For this review, take the finished solid that the model builds, in its own axes (mm). A direction names the side the tool comes from. Round coordinates to 2 decimals unless told otherwise and drop trailing zeros. Write each loop counter-clockwise with the first axis right and the second up, starting at its lowest first coordinate (ties: lowest second). Pieces come first, ordered by that corner, then holes. Notation, with made-up numbers: M -21,34.25 L 9,34.25 A21 ccw 9,71.25 Z; hole C 73,33 d7. An arc over 180 degrees is marked long. Answer in a Markdown table with one row per item.
```python
from build123d import *

# Parameters (mm, degrees)
F0_R           = 38.1
F0_W           = 17.78
F0_H           = 38.1
F2_DEPTH       = 2.54
F3_D           = 3.175
F3_CSINK_D     = 6.858
F3_CSINK_ANGLE = 90
F4_W           = 25.4
F4_H           = 44.45
F4_W_2         = 17.78
F4_H_2         = 38.1
F5_DEPTH       = 1.27


with BuildPart() as f2:
    # F0 (on Top) → F2 (new body)
    with BuildSketch(Plane.XY):
        Circle(F0_R)
        Rectangle(F0_W, F0_H, mode=Mode.SUBTRACT)
    extrude(amount=F2_DEPTH)

    # F3 (through all)
    with Locations(Plane(origin=(0, 0, 0), x_dir=(1, 0, 0), z_dir=(0, 0, -1))):
        with Locations((0, 35.4584), (0, -35.4463979602)):
            CounterSinkHole(F3_D / 2, F3_CSINK_D / 2, counter_sink_angle=F3_CSINK_ANGLE)

    # F4 (on face) → F5 (cut)
    with BuildSketch(Plane.XY.offset(2.54)):
        Rectangle(F4_W, F4_H)
        Rectangle(F4_W_2, F4_H_2, mode=Mode.SUBTRACT)
    extrude(amount=-F5_DEPTH, mode=Mode.SUBTRACT)


solid = f2.part
```
Q1. Mouldability with a two-part tool opening along X and no side actions: class faces 3 (the face through (0.408, -33.622, 1.547)), 4 (the face through (-30.235, -23.183, 1.252)), 5 (the face through (16, 1, 0)) as +X half, -X half, draft (parallel to the pull), parting line (faces both ways), or undercut.
Found:
| item | result |
|---|---|
| face 3 | undercut |
| face 4 | parting line |
| face 5 | draft |
Q2. Take a section at D-D (y = -20.5). State the section outline as (x, z) points, then the cut area to 3 significant figures.
Found:
| item | result |
|---|---|
| outline | M -32.11,0 L 32.11,0 L 32.11,2.54 L 12.7,2.54 L 12.7,1.27 L -12.7,1.27 L -12.7,2.54 L -32.11,2.54 Z |
| area | 131 mm² |
Q3. Machinability: for faces 1 (the face through (11, 0, 1.27)), 2 (the face through (0.24, 33.58, 1.55)), which of the approach directions +Z, -Z, +X, -X, +Y, -Y give a long, thin tool a straight path to every point of the face, cutting with its end or side? Answer none if there is none.
Found:
| item | result |
|---|---|
| face 1 | +Z |
| face 2 | -Z |
Q4. Take a section at B-B (x = 0). State how many separate pieces and enclosed holes the cut face has, then the cut area to 3 significant figures.
Found:
| item | result |
|---|---|
| separate pieces | 4 |
| enclosed holes | 0 |
| area | 66.4 mm² |
Q5. For probe 1 along Y at (x, z) = (0, 2) (3 decimals); probe 2 along X at (y, z) = (0.5, 0.2); probe 3 along X at (y, z) = (1, 1.65), list the stretches that pass through material, from the lowest coordinate up.
Found:
| item | result |
|---|---|
| probe 1 | -38.1 to -37.046, -33.871 to -22.225, 22.225 to 33.859, 37.034 to 38.1 |
| probe 2 | -38.1 to -8.89, 8.89 to 38.1 |
| probe 3 | -38.09 to -12.7, 12.7 to 38.09 |
Q6. Take a section at C-C (z = 0.5). State the section outline as (x, y) points.
Found:
| item | result |
|---|---|
| outline | M -1.31,-38.08 A2.93 cw long 1.31,-38.08 A38.1 ccw 1.29,38.08 A2.93 cw long -1.29,38.08 A38.1 ccw Z; hole M -8.89,-19.05 L 8.89,-19.05 L 8.89,19.05 L -8.89,19.05 Z |
Q7. Take a section at A-A (y = 0). State the section outline as (x, z) points.
Found:
| item | result |
|---|---|
| outline | M -38.1,0 L -8.89,0 L -8.89,1.27 L -12.7,1.27 L -12.7,2.54 L -38.1,2.54 Z; M 8.89,0 L 38.1,0 L 38.1,2.54 L 12.7,2.54 L 12.7,1.27 L 8.89,1.27 Z |
Q8. Insertion check: P1, Ø1.4, axis at y = 5, z = 1, coming from the +X side; P2, Ø1.4, axis at y = 4.5, z = 2, coming from the -X side; P3, Ø1.9, axis at x = 0, y = -35.46, coming from the -Z side; P4, Ø1.4, axis at x = 3.5, z = 0.5, coming from the -Y side. Each pin has a flat end and moves straight along its axis. Give the tip position at first contact, or say it passes through.
Found:
| item | result |
|---|---|
| P1 | x = 37.86 |
| P2 | x = -37.91 |
| P3 | through |
| P4 | y = -38 |
